The listing builds one solid part. Answer for the finished solid, in the listing's coordinates (mm). A direction names the side the tool comes from. Round coordinates to 2 decimals unless told otherwise and drop trailing zeros. Write each loop counter-clockwise with the first axis right and the second up, starting at its lowest first coordinate (ties: lowest second). Pieces come first, ordered by that corner, then holes. Notation, with made-up numbers: (-37, 38) -> (0, 38) arc R18 ccw to (0, 63) -> close; hole circle Ø10 at (42, 76.25). An arc over 180 degrees is marked (long way). Write each question's results on one line, items separated by ' | '. Start each with the question number.
```python
from build123d import *

# Parameters (mm, degrees)
BOSS_EXTRUDE1_DEPTH = 6
SKETCH1_3_R         = 2
BOSS_EXTRUDE2_DEPTH = 27.25
SKETCH2_OUTSIDE_W   = 76.14
SKETCH2_OUTSIDE_H   = 74.8
SKETCH2_OUTSIDE_R   = 4.330127019
CUT_EXTRUDE5_DEPTH  = 29.041264237
CUT_EXTRUDE5_DRAFT  = -45
CHAMFER1_SIZE       = 0.2
SKETCH3_OUTSIDE_W   = 64.57
SKETCH3_OUTSIDE_H   = 63.23
SKETCH3_OUTSIDE_R   = 4.330127019
CUT_EXTRUDE6_DEPTH  = 23.255617268
CUT_EXTRUDE6_DRAFT  = -45


with BuildPart() as part:
    # Sketch1 → Boss-Extrude1 (new body)
    with BuildSketch(Plane(origin=(0, 0, 0), x_dir=(1, 0, 0), z_dir=(0, 1, 0))):
        Polygon((-2.5, -4.330127019), (2.5, -4.330127019), (5, 0), (2.5, 4.330127019), (-2.5, 4.330127019), (-5, 0), align=None)
    extrude(amount=BOSS_EXTRUDE1_DEPTH)

    # Sketch1_3 → Boss-Extrude2 (add)
    with BuildSketch(Plane(origin=(0, 0, 0), x_dir=(1, 0, 0), z_dir=(0, 1, 0))):
        with Locations(Location((0, 0, 0), (0, 0, 270))):
            Circle(SKETCH1_3_R)
    extrude(amount=BOSS_EXTRUDE2_DEPTH)


with BuildPart() as cut_extrude5_tool:
    # Sketch2 outside → Cut-Extrude5 (with draft: the straight prism first)
    with BuildSketch(Plane.XZ):
        Rectangle(SKETCH2_OUTSIDE_W, SKETCH2_OUTSIDE_H)
        Circle(SKETCH2_OUTSIDE_R, mode=Mode.SUBTRACT)
    extrude(amount=-CUT_EXTRUDE5_DEPTH)
    # Cut-Extrude5: the draft: its side faces are tilted about the plane it starts from
    cut_extrude5_sides = [cut_extrude5_tool.faces().sort_by_distance(p)[0] for p in [
        (0, 14.520632118, -37.4),
        (38.07, 14.520632118, 0),
        (0, 14.520632118, 37.4),
        (-38.07, 14.520632118, 0),
        (-4.330127019, 14.520632118, 0),
    ]]
    draft(cut_extrude5_sides, Plane.XZ, CUT_EXTRUDE5_DRAFT)


with BuildPart() as part_1:
    add(part.part)

    # Cut-Extrude5: cut by cut_extrude5_tool
    add(cut_extrude5_tool.part, mode=Mode.SUBTRACT)

    # Chamfer1
    chamfer1_edges = [part_1.edges().sort_by_distance(p)[0] for p in [
        (0, 27.25, -2),
    ]]
    chamfer(chamfer1_edges, length=CHAMFER1_SIZE)


with BuildPart() as cut_extrude6_tool:
    # Sketch3 outside → Cut-Extrude6 (with draft: the straight prism first)
    with BuildSketch(Plane(origin=(0, 6, 0), x_dir=(1, 0, 0), z_dir=(0, 1, 0))):
        Rectangle(SKETCH3_OUTSIDE_W, SKETCH3_OUTSIDE_H)
        Circle(SKETCH3_OUTSIDE_R, mode=Mode.SUBTRACT)
    extrude(amount=-CUT_EXTRUDE6_DEPTH)
    # Cut-Extrude6: the draft: its side faces are tilted about the plane it starts from
    cut_extrude6_sides = [cut_extrude6_tool.faces().sort_by_distance(p)[0] for p in [
        (0, -5.627808634, 31.615),
        (32.285, -5.627808634, 0),
        (0, -5.627808634, -31.615),
        (-32.285, -5.627808634, 0),
        (-4.330127019, -5.627808634, 0),
    ]]
    draft(cut_extrude6_sides, Plane(origin=(0, 6, 0), x_dir=(1, 0, 0), z_dir=(0, 1, 0)), CUT_EXTRUDE6_DRAFT)


with BuildPart() as part_2:
    add(part_1.part)

    # Cut-Extrude6: cut by cut_extrude6_tool
    add(cut_extrude6_tool.part, mode=Mode.SUBTRACT)


solid = part_2.part
```
Q1. The part is cut by section A-A, the plane y = 14.5. Write down the section's boundary in (x, z).
Q2. Find the intervals of material crossed by line 1 (Y direction, x = -3.5, z = 2.5); line 2 (X direction, y = 14.75, z = 0); line 3 (Z direction, x = -1.5, y = 13.5), in increasing order.
Q3. For faces 1 (the conical face through (2.3, 0.2, 3.9)), 2 (the cylindrical face through (-2, 16, 0)), determine the directions among +Z, -Z, +X, -X, +Y, -Y from which every point of the face is accessible in a straight line to the end or side of a thin tool.
Q4. Each of these flat-tipped pins is pushed along its axis until it touches: pin 1 (3 mm diameter, centred on x = -2.5, y = 9, fed in from +Z); pin 2 (4 mm diameter, centred on y = 22, z = -3, fed in from -X); pin 3 (4 mm diameter, centred on y = 22, z = 2, fed in from +X). Where does it stop, or does it pass through?
Answers follow:
1) outline: circle Ø4 at (0, 0)
2) line 1: 0 to 6 | line 2: -2 to 2 | line 3: -1.32 to 1.32
3) face 1: +Z, +X, -Y | face 2: +Y
4) pin 1: z = 1.73 | pin 2: x = -1.73 | pin 3: x = 2
